Can you work these out from the drawing? Everything is in mm from the part's minimum corner. A direction names the side the tool comes from. Round coordinates to 2 decimals unless told otherwise and drop trailing zeros. Loops run counter-clockwise (first coordinate to the right, second up) from the corner with the lowest first, then second, coordinate; pieces in that order, holes last. Notation, with made-up numbers: M -36,62.25 L -8,62.25 A11 ccw -8,72.25 Z; hole C 74.25,3.5 d6. An arc over 180 degrees is marked long. Use a Markdown table: item, result.
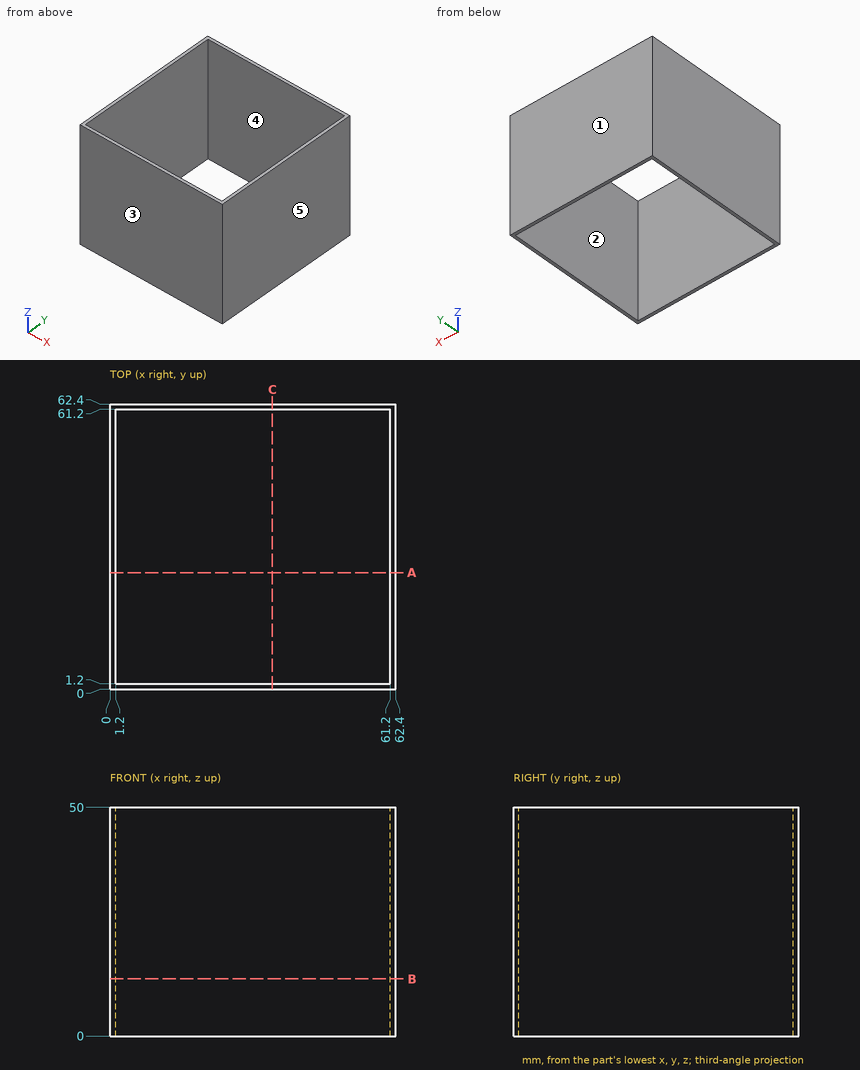
1. We'd pull the mould along X, two halves only. Please class the marked faces 3, 4 and 5: +X half, -X half, draft (parallel to the pull), parting line (faces both ways), or undercut.
Answer sheet:
| item | result |
|---|---|
| face 3 | draft |
| face 4 | undercut |
| face 5 | +X half |
2. I need wall thicknesses on probe 1 along X at (y, z) = (12, 34.5). Which ranges of the line are inside material? Lowest first, please. Write a range as from..to.
Answer sheet:
| item | result |
|---|---|
| probe 1 | 0..1.2, 61.2..62.4 |
3. Which directions (+Z, -Z, +X, -X, +Y, -Y) give clear straight access to the entire face, cutting with the end or side of a thin tool? Please do the marked faces 1 and 2.
Answer sheet:
| item | result |
|---|---|
| face 1 | +Z, -Z, +X, -X, +Y |
| face 2 | +Z, -Z |
4. Imagine slicing it at B-B, the plane z = 12.5. Write out the boundary of the cut face in (x, y).
Answer sheet:
| item | result |
|---|---|
| outline | M 0,0 L 62.4,0 L 62.4,62.4 L 0,62.4 Z; hole M 1.2,1.2 L 61.2,1.2 L 61.2,61.2 L 1.2,61.2 Z |
5. Imagine slicing it at A-A, the plane y = 25.5. Write out the boundary of the cut face in (x, z).
Answer sheet:
| item | result |
|---|---|
| outline | M 0,0 L 1.2,0 L 1.2,50 L 0,50 Z; M 61.2,0 L 62.4,0 L 62.4,50 L 61.2,50 Z |
6. For pin 1 Ø15 at (x, z) = (42.5, 37) entering from -Y, with a flat end and sliding along its axis, tell me the tip position at first contact or that it passes through.
Answer sheet:
| item | result |
|---|---|
| pin 1 | y = 0 |
